from build123d import *

# Parameters (mm, degrees)
SKETCH1_W           = 13
SKETCH1_H           = 13
BOSS_EXTRUDE1_DEPTH = 1
SKETCH2_W           = 10.4
SKETCH2_H           = 10.4
BOSS_EXTRUDE2_DEPTH = 6
SKETCH3_R           = 4.5
CUT_EXTRUDE1_DEPTH  = 4
SKETCH4_R           = 1.25
CUT_EXTRUDE2_DEPTH  = 11.024968828


with BuildPart() as part:
    # Sketch1 → Boss-Extrude1 (new body)
    with BuildSketch(Plane(origin=(0, 0, 0), x_dir=(1, 0, 0), z_dir=(0, 1, 0))):
        Rectangle(SKETCH1_W, SKETCH1_H)
    extrude(amount=BOSS_EXTRUDE1_DEPTH)

    # Sketch2 → Boss-Extrude2 (add)
    with BuildSketch(Plane(origin=(0, 1, 0), x_dir=(1, 0, 0), z_dir=(0, 1, 0))):
        Rectangle(SKETCH2_W, SKETCH2_H)
    extrude(amount=BOSS_EXTRUDE2_DEPTH)

    # Sketch3 → Cut-Extrude1 (cut)
    with BuildSketch(Plane.XZ):
        with Locations(Location((0, 0, 0), (0, 0, 270))):
            Circle(SKETCH3_R)
    extrude(amount=-CUT_EXTRUDE1_DEPTH, mode=Mode.SUBTRACT)

    # Sketch4 → Cut-Extrude2 (cut, through all)
    with BuildSketch(Plane.XZ.offset(-4)):
        with Locations(Location((0, 0, 0), (0, 0, 270))):
            Circle(SKETCH4_R)
    extrude(amount=-CUT_EXTRUDE2_DEPTH, mode=Mode.SUBTRACT)


solid = part.part
The model under review builds one solid part; all positions refer to its coordinate system, in mm. A direction names the side the tool comes from. Round coordinates to 2 decimals unless told otherwise and drop trailing zeros. Write each loop counter-clockwise with the first axis right and the second up, starting at its lowest first coordinate (ties: lowest second). Pieces come first, ordered by that corner, then holes. Notation, with made-up numbers: M 0,47 L 27,47 A30 cw 27,82 Z; hole C 0,75.5 d3. An arc over 180 degrees is marked long. Use a Markdown table: item, result. Add a question column.
Q1. We need section A-A, the plane z = 0. State the section outline as (x, y) points.
Q2. We need section C-C, the plane y = 6.25. State the section outline as (x, z) points, plus the area to 3 significant figures.
Q3. We need section D-D, the plane z = 4.25. State the section outline as (x, y) points, plus the area to 3 significant figures.
Q4. We need section B-B, the plane x = 0. State the section outline as (y, z) points, plus the area to 3 significant figures.
Q5. Machinability: for faces 5 (the face through (5.2, 4, 0)), 6 (the face through (-5.2, 4, 0)), 7 (the face through (1.352, 1.972, -4.292)), which of the approach directions +Z, -Z, +X, -X, +Y, -Y give a long, thin tool a straight path to every point of the face, cutting with its end or side? Answer none if there is none.
Q6. To check wall thickness, follow line 1 (X direction, y = 1.9, z = 0); line 2 (X direction, y = 5.3, z = 0); line 3 (Z direction, x = 1, y = 5.5). State the ranges of each line that lie inside material, in increasing order.
Q7. The part is to be moulded in two halves that separate along Z. For faces 1 (the face through (-1, 4, -1)), 2 (the face through (0, 4, -5.2)), 3 (the face through (0, 4, 5.2)), 4 (the face through (-1.22, 5.48, 0.27)), say which applies: pulls with the +Z half, pulls with the -Z half, needs draft (parallel to the pull), parting line crosses it, or undercut.
Q8. Insertion check: pin 1 (2 mm diameter, centred on x = -4.5, y = 3.5, fed in from -Z); pin 2 (3 mm diameter, centred on y = 5, z = -0.5, fed in from +X); pin 3 (1.8 mm diameter, centred on y = 2.5, z = -2, fed in from -X). Each pin has a flat end and moves straight along its axis. Give the tip position at first contact, or say it passes through.
Findings below:
| question | item | result |
|---|---|---|
| 1 | outline | M -6.5,0 L -4.5,0 L -4.5,4 L -1.25,4 L -1.25,7 L -5.2,7 L -5.2,1 L -6.5,1 Z; M 1.25,4 L 4.5,4 L 4.5,0 L 6.5,0 L 6.5,1 L 5.2,1 L 5.2,7 L 1.25,7 Z |
| 2 | outline | M -5.2,-5.2 L 5.2,-5.2 L 5.2,5.2 L -5.2,5.2 Z; hole C 0,0 d2.5 |
| 2 | area | 103 mm² |
| 3 | outline | M -6.5,0 L -1.48,0 L -1.48,4 L 1.48,4 L 1.48,0 L 6.5,0 L 6.5,1 L 5.2,1 L 5.2,7 L -5.2,7 L -5.2,1 L -6.5,1 Z |
| 3 | area | 63.6 mm² |
| 4 | outline | M 0,-6.5 L 1,-6.5 L 1,-5.2 L 7,-5.2 L 7,-1.25 L 4,-1.25 L 4,-4.5 L 0,-4.5 Z; M 0,4.5 L 4,4.5 L 4,1.25 L 7,1.25 L 7,5.2 L 1,5.2 L 1,6.5 L 0,6.5 Z |
| 4 | area | 31.9 mm² |
| 5 | face 5 | +Z, -Z, +X, +Y |
| 5 | face 6 | +Z, -Z, -X, +Y |
| 5 | face 7 | -Y |
| 6 | line 1 | x = -5.2 to -4.5, 4.5 to 5.2 |
| 6 | line 2 | x = -5.2 to -1.25, 1.25 to 5.2 |
| 6 | line 3 | z = -5.2 to -0.75, 0.75 to 5.2 |
| 7 | face 1 | undercut |
| 7 | face 2 | pulls with the -Z half |
| 7 | face 3 | pulls with the +Z half |
| 7 | face 4 | undercut |
| 8 | pin 1 | stops at z = -5.2 |
| 8 | pin 2 | stops at x = 5.2 |
| 8 | pin 3 | stops at x = -5.2 |
